Read the model definition and answer for the solid it produces. Units are mm, in the model's axes. Face numbers are marked on the shaded views. A direction names the side the tool comes from. Coordinates: 2 decimals unless noted, no trailing zeros. Write each loop counter-clockwise with the first axis right and the second up, starting at its lowest first coordinate (ties: lowest second). Pieces come first, ordered by that corner, then holes.
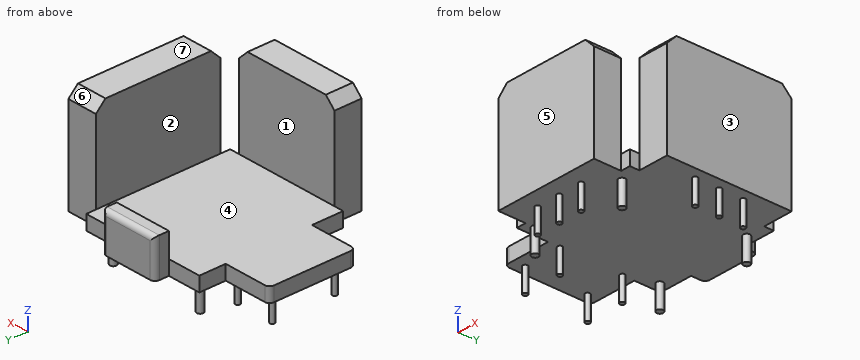
from build123d import *

# Parameters (mm, degrees)
RESSALTO_EXTRUS_O4_DEPTH  = 1.5
ESBO_O5_W                 = 6
ESBO_O5_H                 = 1.5
RESSALTO_EXTRUS_O6_DEPTH  = 4
RESSALTO_EXTRUS_O7_DEPTH  = 11
ESBO_O8_W                 = 2.01
ESBO_O8_H                 = 1.51
RESSALTO_EXTRUS_O15_DEPTH = 11
ESBO_O9_W                 = 1.51
ESBO_O9_H                 = 2.01
RESSALTO_EXTRUS_O16_DEPTH = 11
ESBO_O10_R                = 0.25
RESSALTO_EXTRUS_O17_DEPTH = 2.5
ESBO_O11_R                = 0.35
RESSALTO_EXTRUS_O18_DEPTH = 4
ESBO_O12_R                = 0.25
RESSALTO_EXTRUS_O19_DEPTH = 2.5
CHANFRO1_SIZE             = 1
FILETE2_R                 = 0.5


with BuildPart() as part:
    # Esboço3 → Ressalto-extrusão4 (new body)
    with BuildSketch(Plane(origin=(0, 0, 0), x_dir=(-1, 0, 0), z_dir=(0, 0, -1))):
        Polygon((11.5, 4.75), (6.5, 4.75), (6.5, 7.5), (-6.5, 7.5), (-6.5, 6.5), (-8.5, 6.5), (-8.5, 5), (-6.5, 5), (-6.5, -5), (-8.5, -5), (-8.5, -6.5), (-6.5, -6.5), (-6.5, -7.5), (-5.5, -7.5), (-5.5, -9.5), (-4, -9.5), (-4, -7.5), (4, -7.5), (4, -9.5), (5.5, -9.5), (5.5, -7.5), (6.5, -7.5), (6.5, -4.25), (11.5, -4.25), align=None)
    extrude(amount=RESSALTO_EXTRUS_O4_DEPTH)

    # Esboço5 → Ressalto-extrusão6 (add)
    with BuildSketch(Plane(origin=(0, 0, -1.5), x_dir=(-1, 0, 0), z_dir=(0, 0, -1))):
        with Locations((0, 8.25)):
            Rectangle(ESBO_O5_W, ESBO_O5_H)
    extrude(amount=-RESSALTO_EXTRUS_O6_DEPTH)

    # Esboço6 → Ressalto-extrusão7 (add)
    with BuildSketch(Plane(origin=(0, 0, -1.5), x_dir=(-1, 0, 0), z_dir=(0, 0, -1))):
        Polygon((-6.5, 4.99), (-8.51, 4.99), (-8.51, 6.5), (-9.663134603, 6.5), (-9.663134603, -6.5), (-8.51, -6.5), (-8.51, -4.99), (-6.5, -4.99), align=None)
        Polygon((-3.99, -7.5), (-3.99, -9.51), (-5.5, -9.51), (-5.5, -10.329816926), (5.5, -10.329816926), (5.5, -9.51), (3.99, -9.51), (3.99, -7.5), align=None)
    extrude(amount=-RESSALTO_EXTRUS_O7_DEPTH)

    # Esboço8 → Ressalto-extrusão15 (add)
    with BuildSketch(Plane.XY.offset(9.5)):
        with Locations((7.505, -5.745)):
            Rectangle(ESBO_O8_W, ESBO_O8_H)
        with Locations((7.505, 5.745)):
            Rectangle(ESBO_O8_W, ESBO_O8_H)
    extrude(amount=-RESSALTO_EXTRUS_O15_DEPTH)

    # Esboço9 → Ressalto-extrusão16 (add)
    with BuildSketch(Plane.XY.offset(9.5)):
        with Locations((-4.745, -8.505)):
            Rectangle(ESBO_O9_W, ESBO_O9_H)
        with Locations((4.745, -8.505)):
            Rectangle(ESBO_O9_W, ESBO_O9_H)
    extrude(amount=-RESSALTO_EXTRUS_O16_DEPTH)

    # Esboço10 → Ressalto-extrusão17 (add)
    with BuildSketch(Plane(origin=(0, 0, -1.5), x_dir=(-1, 0, 0), z_dir=(0, 0, -1))):
        with Locations((10.5, 3.5)):
            Circle(ESBO_O10_R)
        with Locations((6.5, 3.5)):
            Circle(ESBO_O10_R)
        with Locations((10.5, -3)):
            Circle(ESBO_O10_R)
        with Locations((6.5, -3)):
            Circle(ESBO_O10_R)
    extrude(amount=RESSALTO_EXTRUS_O17_DEPTH)

    # Esboço11 → Ressalto-extrusão18 (add)
    with BuildSketch(Plane.XY):
        with Locations((-5.5, 6.5)):
            Circle(ESBO_O11_R)
        with Locations((4.5, 6.5)):
            Circle(ESBO_O11_R)
        with Locations((4.5, -6.5)):
            Circle(ESBO_O11_R)
        with Locations((-5.5, -6.5)):
            Circle(ESBO_O11_R)
    extrude(amount=-RESSALTO_EXTRUS_O18_DEPTH)

    # Esboço12 → Ressalto-extrusão19 (add)
    with BuildSketch(Plane(origin=(0, 0, -1.5), x_dir=(-1, 0, 0), z_dir=(0, 0, -1))):
        with Locations((3, -8.5)):
            Circle(ESBO_O12_R)
        with Locations((0.5, -8.5)):
            Circle(ESBO_O12_R)
        with Locations((-2, -8.5)):
            Circle(ESBO_O12_R)
        with Locations((-8.5, -2.5)):
            Circle(ESBO_O12_R)
        with Locations((-8.5, 0)):
            Circle(ESBO_O12_R)
        with Locations((-8.5, 2.5)):
            Circle(ESBO_O12_R)
    extrude(amount=RESSALTO_EXTRUS_O19_DEPTH)

    # Chanfro1
    chanfro1_edges = [part.edges().sort_by_distance(p)[0] for p in [
        (-5.5, -8.914908463, 9.5),
        (5.5, -8.914908463, 9.5),
        (8.081567302, -6.5, 9.5),
        (8.081567302, 6.5, 9.5),
    ]]
    chamfer(chanfro1_edges, length=CHANFRO1_SIZE)

    # Filete2
    filete2_edges = [part.edges().sort_by_distance(p)[0] for p in [
        (-11.5, 4.75, -0.75),
        (-11.5, -4.25, -0.75),
        (-3, 9, 0.5),
        (0, 9, 2.5),
        (3, 9, 0.5),
    ]]
    fillet(filete2_edges, radius=FILETE2_R)


solid = part.part
Item 1: The part is cut by section A-A (z = 6.5). Give the vertices of the cut face in (x, y), and give its area (3 significant figures).
Item 2: Determine the mould class of the marked faces 4, 5, 6 and 7 for opening direction Y: +Y half, -Y half, draft (parallel to the pull), parting line (faces both ways), or undercut.
Item 3: The part is cut by section B-B (z = -2). State how many separate pieces and enclosed holes the cut face has, and give its area (3 significant figures).
Item 4: Given pin 1 (1.2 mm diameter, centred on x = -4, z = -0.5, fed in from +Y); pin 2 (3 mm diameter, centred on y = -9, z = 1.5, fed in from +X); pin 3 (0.8 mm diameter, centred on y = -5, z = -0.5, fed in from -X), each flat-ended and moving along its own axis, determine where each tip first touches the part or whether it passes through.
Item 5: Find the intervals of material crossed by probe 1 along Y at (x, z) = (-0.75, 0.5); probe 2 along Z at (x, y) = (-3.25, -1); probe 3 along X at (y, z) = (-1.5, 3.5), in increasing order.
Item 6: The part is cut by section C-C (x = 3.5). Give the vertices of the cut face in (y, z), and give its area (3 significant figures).
Item 7: The part is cut by section D-D (x = -8.5). Give the vertices of the cut face in (y, z), and give its area (3 significant figures).
Item 8: For the marked faces 1, 2 and 3, determine the directions among +Z, -Z, +X, -X, +Y, -Y from which every point of the face is accessible in a straight line to the end or side of a thin tool.
Answer:
1. outline: (-5.5, -10.33) - (5.5, -10.33) - (5.5, -7.5) - (-5.5, -7.5) - close; (6.5, -6.5) - (9.66, -6.5) - (9.66, 6.5) - (6.5, 6.5) - close
1. area: 72.2 mm2
2. face 4: undercut
2. face 5: -Y half
2. face 6: +Y half
2. face 7: draft
3. separate pieces: 14
3. enclosed holes: 0
3. area: 3.50 mm2
4. pin 1: stops at y = 7.5
4. pin 2: stops at x = 5.5
4. pin 3: stops at x = -6.5
5. probe 1: y = -10.33 to -7.5, 7.5 to 9
5. probe 2: z = -1.5 to 0
5. probe 3: x = 6.5 to 9.66
6. outline: (-10.33, -1.5) - (7.5, -1.5) - (7.5, 0) - (-7.5, 0) - (-7.5, 9.5) - (-10.33, 9.5) - close
6. area: 53.6 mm2
7. outline: (-4.25, -1.5) - (4.75, -1.5) - (4.75, 0) - (-4.25, 0) - close
7. area: 13.5 mm2
8. face 1: +Z, +X, -X
8. face 2: +Z, -X, +Y, -Y
8. face 3: +Z, -Z, +X, +Y, -Y
